Verification items for the finished model (mm, model axes). A direction names the side the tool comes from. Round coordinates to 2 decimals unless told otherwise and drop trailing zeros. Order: outer loops, then holes, each group sorted by start corner. A loop starts at its lowest first (then second) coordinate and runs counter-clockwise, first axis right, second up. Notation, with made-up numbers: M 42,-16.75 L 59,-16.75 A19 ccw 59,15.25 Z; hole C -6.75,72.25 d7. An arc over 180 degrees is marked long. Return JSON: item names as keys, results as strings. Group by question number.
from build123d import *

# Parameters (mm, degrees)
CUT_EXTRUDE1_DEPTH      = 90.543285622
CUT_EXTRUDE1_DEPTH_BACK = 90.543285622
SKETCH3_W               = 20
SKETCH3_H               = 28
SHELL1_START            = -60
SHELL1_DEPTH            = 50
SHELL1_START_2          = -17
SHELL1_2_DEPTH          = 7
SHELL1_3_DEPTH          = 28
SKETCH4_R               = 41
BOSS_EXTRUDE2_DEPTH     = 18
CUT_EXTRUDE2_DEPTH      = 107.579782323
CUT_EXTRUDE2_DEPTH_BACK = 107.579782323
SKETCH5_R               = 5


# Read off the part's stored shape, not the designer's step: Shell1
with BuildPart() as part:
    # Sketch1 → Revolve1 (revolve)
    with BuildSketch(Plane.XY):
        Polygon((0, -60), (0, 0), (-47, 0), (-47, -10), (-45, -10), (-45, -12), (-47, -12), (-47, -15), (-45, -15), (-45, -17), (-47, -17), (-47, -20), (-45, -20), (-45, -22), (-47, -22), (-47, -60), align=None)
    revolve(axis=Axis((0, 0, 0), (0, -1, 0)))

    # Sketch3 → Cut-Extrude1 (cut, two sides: drawn at the far end of the back side and taken through both)
    with BuildSketch(Plane.XY.offset(-CUT_EXTRUDE1_DEPTH_BACK)):
        with Locations((-37.5, -41)):
            Rectangle(SKETCH3_W, SKETCH3_H)
        with Locations((37.5, -41)):
            Rectangle(SKETCH3_W, SKETCH3_H)
    extrude(amount=CUT_EXTRUDE1_DEPTH + CUT_EXTRUDE1_DEPTH_BACK, mode=Mode.SUBTRACT)

    # Shell1 outline → Shell1 (cut)
    with BuildSketch(Plane(origin=(0, 0, 0), x_dir=(1, 0, 0), z_dir=(0, 1, 0)).offset(SHELL1_START)):
        with BuildLine():
            Line((17.5, -30.310889132), (17.5, 30.310889132))
            ThreePointArc((17.5, 30.310889132), (0, 35), (-17.5, 30.310889132))
            Line((-17.5, 30.310889132), (-17.5, -30.310889132))
            ThreePointArc((-17.5, -30.310889132), (0, -35), (17.5, -30.310889132))
        make_face()
    extrude(amount=SHELL1_DEPTH, mode=Mode.SUBTRACT)

    # Shell1 2 outline → Shell1 2 (cut)
    with BuildSketch(Plane(origin=(0, 0, 0), x_dir=(1, 0, 0), z_dir=(0, 1, 0)).offset(SHELL1_START_2)):
        with BuildLine():
            ThreePointArc((17.5, -30.310889132), (35, 0), (17.5, 30.310889132))
            Line((17.5, 30.310889132), (17.5, -30.310889132))
        make_face()
        with BuildLine():
            Line((-17.5, -30.310889132), (-17.5, 30.310889132))
            ThreePointArc((-17.5, 30.310889132), (-35, 0), (-17.5, -30.310889132))
        make_face()
    extrude(amount=SHELL1_2_DEPTH, mode=Mode.SUBTRACT)

    # Shell1 3 outline → Shell1 3 (cut)
    with BuildSketch(Plane(origin=(0, 0, 0), x_dir=(1, 0, 0), z_dir=(0, 1, 0)).offset(SHELL1_START)):
        with BuildLine():
            Line((17.5, 30.310889132), (17.5, 32.599846625))
            ThreePointArc((17.5, 32.599846625), (0, 37), (-17.5, 32.599846625))
            Line((-17.5, 32.599846625), (-17.5, 30.310889132))
            ThreePointArc((-17.5, 30.310889132), (0, 35), (17.5, 30.310889132))
        make_face()
        with BuildLine():
            Line((17.5, -32.599846625), (17.5, -30.310889132))
            ThreePointArc((17.5, -30.310889132), (0, -35), (-17.5, -30.310889132))
            Line((-17.5, -30.310889132), (-17.5, -32.599846625))
            ThreePointArc((-17.5, -32.599846625), (0, -37), (17.5, -32.599846625))
        make_face()
    extrude(amount=SHELL1_3_DEPTH, mode=Mode.SUBTRACT)

    # Sketch4 → Boss-Extrude2 (add)
    with BuildSketch(Plane(origin=(0, 0, 0), x_dir=(1, 0, 0), z_dir=(0, 1, 0))):
        Circle(SKETCH4_R)
    extrude(amount=-BOSS_EXTRUDE2_DEPTH)

    # Sketch5 → Cut-Extrude2 (cut, two sides: drawn at the far end of the back side and taken through both)
    with BuildSketch(Plane(origin=(27.5, 0, 0), x_dir=(0, 0, -1), z_dir=(1, 0, 0)).offset(-CUT_EXTRUDE2_DEPTH_BACK)):
        with Locations(Location((0, -41, 0), (0, 0, 270))):
            Circle(SKETCH5_R)
    extrude(amount=CUT_EXTRUDE2_DEPTH + CUT_EXTRUDE2_DEPTH_BACK, mode=Mode.SUBTRACT)


solid = part.part
1. Thickness scan on line 1 along Y through (x, z) = (32, 24); line 2 along X through (y, z) = (-44.5, -32.5); line 3 along X through (y, z) = (-21, -17). Record the ranges inside material, lowest first. Write a range as from..to.
2. Draft check along X on faces 4 (the face through (0, -25, 35)), 5 (the face through (-44.83, -18.52, -14.12)), 6 (the face through (35, -27, -1)), 7 (the face through (-27.5, -47, -1)). Enter one of: +X half, -X half, draft (parallel to the pull), parting line (faces both ways), or undercut.
3. Access from +Z, -Z, +X, -X, +Y, -Y to the whole of each face (thin tool, end or side, straight path). Record for faces 1 (the face through (45.04, -12, 3.26)), 2 (the face through (-35, -55, -1)), 3 (the face through (-17.5, -35, 0)).
4. Cross-section at B-B (y = -25). Enter the section's corners in (x, z).
5. Go/stop test with flat-tipped pins: pin 1 (3 mm diameter, centred on x = -9, y = -34, fed in from -Z); pin 2 (10 mm diameter, centred on x = 34.5, z = -16.5, fed in from +Y); pin 3 (1.5 mm diameter, centred on y = -31.5, z = -13, fed in from -X); pin 4 (7.5 mm diameter, centred on x = 4, z = 32.5, fed in from -Y). Record where each tip stops, or that it passes through.
6. Cross-section at A-A (y = -38). Enter the section's corners in (x, z).
Computed:
{
 "1": {"line 1": "y = -60..-55, -27..0", "line 2": "x = -27.5..-17.5, 17.5..27.5", "line 3": "x = -41.67..-17.5, 17.5..41.67"},
 "2": {"face 4": "undercut", "face 5": "parting line", "face 6": "draft", "face 7": "-X half"},
 "3": {"face 1": "none", "face 2": "+Z, -Z, -X", "face 3": "-Y"},
 "4": {"outline": "C 0,0 d94; hole M -17.5,-30.31 A35 ccw 17.5,-30.31 L 17.5,30.31 A35 ccw -17.5,30.31 Z"},
 "5": {"pin 1": "stops at z = -46.4", "pin 2": "stops at y = 0", "pin 3": "stops at x = -27.5", "pin 4": "stops at y = -32"},
 "6": {"outline": "M -27.5,-38.11 A47 ccw 27.5,-38.11 L 27.5,-4 L 17.5,-4 L 17.5,-32.6 A37 cw -17.5,-32.6 L -17.5,-4 L -27.5,-4 Z; M -27.5,4 L -17.5,4 L -17.5,32.6 A37 cw 17.5,32.6 L 17.5,4 L 27.5,4 L 27.5,38.11 A47 ccw -27.5,38.11 Z"}
}
